Read the model definition and answer for the solid it produces. Units are mm, in the model's axes. A direction names the side the tool comes from. Give positions to 0.01 mm unless a question says otherwise; leave off trailing zeros. Write each loop counter-clockwise with the first axis right and the second up, starting at its lowest first coordinate (ties: lowest second). Pieces come first, ordered by that corner, then holes. Notation, with made-up numbers: (-23.75, 86) -> (11.25, 86) arc R28 cw to (11.25, 108) -> close; hole circle Ø1 at (13.5, 31.25). An arc over 180 degrees is marked (long way). Use a Markdown table: item, result.
from build123d import *

# Parameters (mm, degrees)
PAD_DEPTH       = 6
SKETCH001_R     = 1.3
POCKET_DEPTH    = 9
SKETCH002_R     = 1.3
POCKET001_DEPTH = 13.001


with BuildPart() as part:
    # Sketch → Pad (new body)
    with BuildSketch(Plane.XY):
        Polygon((-7, -1.6), (0, -1.6), (0, 0), (9, 0), (9, 11.4), (-2, 11.4), (-7, 6.4), align=None)
    extrude(amount=PAD_DEPTH)

    # Sketch001 → Pocket (cut)
    with BuildSketch(Plane(origin=(-7, 0, 0), x_dir=(0, -1, 0), z_dir=(-1, 0, 0))):
        with Locations((-2.4, 3)):
            Circle(SKETCH001_R)
    extrude(amount=-POCKET_DEPTH, mode=Mode.SUBTRACT)

    # Sketch002 → Pocket001 (cut, through all)
    with BuildSketch(Plane(origin=(0, 11.4, 0), x_dir=(-1, 0, 0), z_dir=(0, 1, 0))):
        with Locations((-4.5, 3)):
            Circle(SKETCH002_R)
    extrude(amount=-POCKET001_DEPTH, mode=Mode.SUBTRACT)


solid = part.part
Item 1: A tool of negligible diameter and unlimited length cuts with its end or side. For faces 1 (the face through (2, 2, 3)), 2 (the face through (1, 5, 0)), 3 (the face through (0, -1, 3)), from which of +Z, -Z, +X, -X, +Y, -Y can it reach the whole face along a straight path? Write none if from no direction.
Return value:
| item | result |
|---|---|
| face 1 | -X |
| face 2 | -Z, +X, -X, +Y, -Y |
| face 3 | +Z, -Z, +X, -Y |
Item 2: A cutting plane is placed at C-C (y = 2.4). Give the vertices of the cut face in (x, z).
Return value:
| item | result |
|---|---|
| outline | (-7, 0) -> (9, 0) -> (9, 6) -> (-7, 6) -> (-7, 4.3) -> (2, 4.3) -> (2, 1.7) -> (-7, 1.7) -> close; hole circle Ø2.6 at (4.5, 3) |
Item 3: Each of these flat-tipped pins is pushed along its axis until it touches: P1, Ø5, axis at x = -2, y = 5.5, coming from the -Z side; P2, Ø1.8, axis at y = -1, z = 4, coming from the +X side; P3, Ø1, axis at y = 8.5, z = 4, coming from the -X side; P4, Ø1, axis at x = -4.5, z = 5, coming from the +Y side. Where does it stop, or does it pass through?
Return value:
| item | result |
|---|---|
| P1 | z = 0 |
| P2 | x = 0 |
| P3 | x = -5.4 |
| P4 | y = 9.4 |
Item 4: A cutting plane is placed at D-D (x = 1.25). Give the vertices of the cut face in (y, z), then the cut area to 3 significant figures.
Return value:
| item | result |
|---|---|
| outline | (0, 0) -> (11.4, 0) -> (11.4, 6) -> (0, 6) -> close; hole circle Ø2.6 at (2.4, 3) |
| area | 63.1 mm^2 |
Item 5: Straight lines are drawn through the part: line 1 along Z through (x, y) = (-2.5, 2.4); line 2 along Y through (x, z) = (-3.5, 2); line 3 along Y through (x, z) = (3.75, 5.15). For each, find the intervals that lie inside material, in ascending order. Write a range as [from, to].
Return value:
| item | result |
|---|---|
| line 1 | [0, 1.7], [4.3, 6] |
| line 2 | [-1.6, 1.57], [3.23, 9.9] |
| line 3 | [0, 11.4] |
Item 6: A cutting plane is placed at B-B (z = 3). Give the vertices of the cut face in (x, y).
Return value:
| item | result |
|---|---|
| outline | (-7, -1.6) -> (0, -1.6) -> (0, 0) -> (3.2, 0) -> (3.2, 11.4) -> (-2, 11.4) -> (-7, 6.4) -> (-7, 3.7) -> (2, 3.7) -> (2, 1.1) -> (-7, 1.1) -> close; (5.8, 0) -> (9, 0) -> (9, 11.4) -> (5.8, 11.4) -> close |
Item 7: For a pull along X with two mould halves and no side action, classify faces 4 (the face through (4.67, 5.78, 4.29)), 5 (the face through (-7, 1.6, 1.6)), 6 (the face through (-4, -1.6, 3)) as +X half, -X half, draft (parallel to the pull), parting line (faces both ways), or undercut.
Return value:
| item | result |
|---|---|
| face 4 | undercut |
| face 5 | -X half |
| face 6 | draft |
Item 8: A cutting plane is placed at A-A (x = 4.5). Give the vertices of the cut face in (y, z).
Return value:
| item | result |
|---|---|
| outline | (0, 0) -> (11.4, 0) -> (11.4, 1.7) -> (0, 1.7) -> close; (0, 4.3) -> (11.4, 4.3) -> (11.4, 6) -> (0, 6) -> close |
